Geometry: final body of the model. Coordinates: model frame, mm. A direction names the side the tool comes from. Give positions to 0.01 mm unless a question says otherwise; leave off trailing zeros. Order: outer loops, then holes, each group sorted by start corner. A loop starts at its lowest first (then second) coordinate and runs counter-clockwise, first axis right, second up. Notation, with made-up numbers: (59.25, 14) -> (114.25, 14) arc R17 cw to (114.25, 41) -> close; hole circle Ø5 at (84.25, 75.5). An arc over 180 degrees is marked (long way). One line per question, with ' | ' between items. Start each with the question number.
(1) Section B-B (z = 4). State how many separate pieces and enclosed holes the cut face has, then the cut area to 3 significant figures.
(2) Set-up query: faces 1 (the face through (-172, 85.24, 3)), 2 (the face through (-172, 147.74, 3)). Return all of +Z, -Z, +X, -X, +Y, -Y with unobstructed straight access to the full face (end or side cutting, diameter ignored); none if empty.
(3) Mould query, pull axis X, two halves, no side actions, for faces 3 (the face through (-258.738, 67.84, 2.958)), 4 (the face through (-267.98, 144.73, 3.04)), 5 (the face through (-70.83, 101, 3)), 6 (the face through (-172, 102, 0)). Classes: +X half, -X half, draft (parallel to the pull), parting line (faces both ways), or undercut.
(4) Section A-A (x = -123). Return loops of the section in (y, z), then the cut area to 3 significant figures.
(5) Ray query, L1, parallel to Y at x = -199.5, z = 4.5; L2, parallel to Y at x = -156, z = 0.75; L3, parallel to Y at x = -115, z = 3.1. Return the intervals inside material, ascending.
```python
from build123d import *

# Parameters (mm, degrees)
SKETCH_1_W          = 200
SKETCH_1_H          = 93
SKETCH_1_W_2        = 160
SKETCH_1_H_2        = 10
EXTRUDE_1_DEPTH     = 6
SKETCH_2_R          = 2
CUT_EXTRUDE_1_DEPTH = 6
FILLET_1_R          = 10


with BuildPart() as part:
    # 草圖1 → 填料-伸長1 (new body)
    with BuildSketch(Plane.XY):
        with Locations((-170.830010195, 101.23957139)):
            Rectangle(SKETCH_1_W, SKETCH_1_H)
        with Locations((-170.830010195, 122.23957139)):
            Rectangle(SKETCH_1_W_2, SKETCH_1_H_2, mode=Mode.SUBTRACT)
        with Locations((-170.830010195, 80.23957139)):
            Rectangle(SKETCH_1_W_2, SKETCH_1_H_2, mode=Mode.SUBTRACT)
    extrude(amount=EXTRUDE_1_DEPTH)

    # 草圖2 → 除料-伸長1 (cut)
    with BuildSketch(Plane(origin=(0, 0, 0), x_dir=(-1, 0, 0), z_dir=(0, 0, -1))):
        with Locations((84.830010195, 135.23957139)):
            Circle(SKETCH_2_R)
        with Locations((113.630010195, 135.23957139)):
            Circle(SKETCH_2_R)
        with Locations((156.430010195, 135.23957139)):
            Circle(SKETCH_2_R)
        with Locations((185.230010195, 135.23957139)):
            Circle(SKETCH_2_R)
        with Locations((228.030010195, 135.23957139)):
            Circle(SKETCH_2_R)
        with Locations((256.830010195, 135.23957139)):
            Circle(SKETCH_2_R)
        with Locations((84.830010195, 67.23957139)):
            Circle(SKETCH_2_R)
        with Locations((113.630010195, 67.23957139)):
            Circle(SKETCH_2_R)
        with Locations((156.430010195, 67.23957139)):
            Circle(SKETCH_2_R)
        with Locations((185.230010195, 67.23957139)):
            Circle(SKETCH_2_R)
        with Locations((228.030010195, 67.23957139)):
            Circle(SKETCH_2_R)
        with Locations((256.830010195, 67.23957139)):
            Circle(SKETCH_2_R)
    extrude(amount=-CUT_EXTRUDE_1_DEPTH, mode=Mode.SUBTRACT)

    # 圓角1
    fillet_1_edges = [part.edges().sort_by_distance(p)[0] for p in [
        (-70.830010195, 54.73957139, 3),
        (-270.830010195, 54.73957139, 3),
        (-270.830010195, 147.73957139, 3),
        (-70.830010195, 147.73957139, 3),
    ]]
    fillet(fillet_1_edges, radius=FILLET_1_R)


solid = part.part
```
Response:
1) separate pieces: 1 | enclosed holes: 14 | area: 15,200 mm^2
2) face 1: +Z, -Z | face 2: +Z, -Z, +X, -X, +Y
3) face 3: undercut | face 4: -X half | face 5: +X half | face 6: draft
4) outline: (54.74, 0) -> (75.24, 0) -> (75.24, 6) -> (54.74, 6) -> close; (85.24, 0) -> (117.24, 0) -> (117.24, 6) -> (85.24, 6) -> close; (127.24, 0) -> (147.74, 0) -> (147.74, 6) -> (127.24, 6) -> close | area: 438 mm^2
5) L1: y = 54.74 to 75.24, 85.24 to 117.24, 127.24 to 147.74 | L2: y = 54.74 to 65.29, 69.19 to 75.24, 85.24 to 117.24, 127.24 to 133.29, 137.19 to 147.74 | L3: y = 54.74 to 65.78, 68.7 to 75.24, 85.24 to 117.24, 127.24 to 133.78, 136.7 to 147.74
